The model under review builds one solid part; all positions refer to its coordinate system, in mm. A direction names the side the tool comes from. Coordinates: 2 decimals unless noted, no trailing zeros. Order: outer loops, then holes, each group sorted by start corner. A loop starts at its lowest first (then second) coordinate and runs counter-clockwise, first axis right, second up. Notation, with made-up numbers: M -2,23 L 31,23 A37 cw 31,59 Z; hole C 24,22 d4. An arc over 180 degrees is marked long. Answer in a Markdown table with one row per item.
from build123d import *

# Parameters (mm, degrees)
SKETCH_1_R      = 17.5
EXTRUDE_1_DEPTH = 30
SKETCH_2_R      = 20
EXTRUDE_2_DEPTH = 75
SKETCH_3_R      = 22
EXTRUDE_3_DEPTH = 20
SKETCH_5_R      = 24
EXTRUDE_4_DEPTH = 12
SKETCH_6_R      = 17.5
EXTRUDE_5_DEPTH = 30


with BuildPart() as part:
    # 草图1 → 凸台-拉伸1 (new body)
    with BuildSketch(Plane(origin=(0, 0, 0), x_dir=(1, 0, 0), z_dir=(0, 1, 0))):
        with Locations(Location((0, 0, 0), (0, 0, 270))):
            Circle(SKETCH_1_R)
    extrude(amount=EXTRUDE_1_DEPTH)

    # 草图2 → 凸台-拉伸2 (add)
    with BuildSketch(Plane(origin=(0, 30, 0), x_dir=(1, 0, 0), z_dir=(0, 1, 0))):
        with Locations(Location((0, 0, 0), (0, 0, 270))):
            Circle(SKETCH_2_R)
    extrude(amount=EXTRUDE_2_DEPTH)

    # 草图3 → 凸台-拉伸3 (add)
    with BuildSketch(Plane(origin=(0, 105, 0), x_dir=(1, 0, 0), z_dir=(0, 1, 0))):
        with Locations(Location((0, 0, 0), (0, 0, 270))):
            Circle(SKETCH_3_R)
    extrude(amount=EXTRUDE_3_DEPTH)

    # 草图5 → 凸台-拉伸4 (add)
    with BuildSketch(Plane(origin=(0, 125, 0), x_dir=(1, 0, 0), z_dir=(0, 1, 0))):
        with Locations(Location((0, 0, 0), (0, 0, 270))):
            Circle(SKETCH_5_R)
    extrude(amount=EXTRUDE_4_DEPTH)

    # 草图6 → 凸台-拉伸5 (add)
    with BuildSketch(Plane(origin=(0, 137, 0), x_dir=(1, 0, 0), z_dir=(0, 1, 0))):
        with Locations(Location((0, 0, 0), (0, 0, 270))):
            Circle(SKETCH_6_R)
    extrude(amount=EXTRUDE_5_DEPTH)


solid = part.part
(1) Insertion check: P1, Ø10, axis at y = 25.5, z = 15, coming from the +X side; P2, Ø4, axis at x = 12.5, y = 90, coming from the +Z side; P3, Ø4, axis at x = 2, y = 26.5, coming from the -Z side. Each pin has a flat end and moves straight along its axis. Give the tip position at first contact, or say it passes through.
Report:
| item | result |
|---|---|
| P1 | x = 15.35 |
| P2 | z = 17.02 |
| P3 | z = -17.5 |
(2) Take a section at C-C (y = 86). Write out the cut boundary in (x, z), then the cut area to 3 significant figures.
Report:
| item | result |
|---|---|
| outline | C 0,0 d40 |
| area | 1,260 mm^2 |
(3) Take a section at B-B (z = 0). Write out the cut boundary in (x, y).
Report:
| item | result |
|---|---|
| outline | M -24,125 L -22,125 L -22,105 L -20,105 L -20,30 L -17.5,30 L -17.5,0 L 17.5,0 L 17.5,30 L 20,30 L 20,105 L 22,105 L 22,125 L 24,125 L 24,137 L 17.5,137 L 17.5,167 L -17.5,167 L -17.5,137 L -24,137 Z |
(4) Take a section at D-D (y = 16). Write out the cut boundary in (x, z), then the cut area to 3 significant figures.
Report:
| item | result |
|---|---|
| outline | C 0,0 d35 |
| area | 962 mm^2 |
(5) Take a section at A-A (x = 0). Write out the cut boundary in (y, z), then the cut area to 3 significant figures.
Report:
| item | result |
|---|---|
| outline | M 0,-17.5 L 30,-17.5 L 30,-20 L 105,-20 L 105,-22 L 125,-22 L 125,-24 L 137,-24 L 137,-17.5 L 167,-17.5 L 167,17.5 L 137,17.5 L 137,24 L 125,24 L 125,22 L 105,22 L 105,20 L 30,20 L 30,17.5 L 0,17.5 Z |
| area | 6,560 mm^2 |
(6) To check wall thickness, follow line 1 (Z direction, x = 1, y = 109.5); line 2 (X direction, y = 71, z = 0); line 3 (Y direction, x = 5, z = -20). State the ranges of each line that lie inside material, in increasing order. Write a range as [from, to].
Report:
| item | result |
|---|---|
| line 1 | [-21.98, 21.98] |
| line 2 | [-20, 20] |
| line 3 | [105, 137] |
(7) Machinability: for faces 1 (the cylindrical face through (7.21, 130.92, 22.89)), 2 (the cylindrical face through (-10.648, 151.79, -13.887)), 3 (the flat face through (-18, 30, 0)), which of the approach directions +Z, -Z, +X, -X, +Y, -Y give a long, thin tool a straight path to every point of the face, cutting with its end or side? Answer none if there is none.
Report:
| item | result |
|---|---|
| face 1 | +Y, -Y |
| face 2 | +Y |
| face 3 | -Y |
